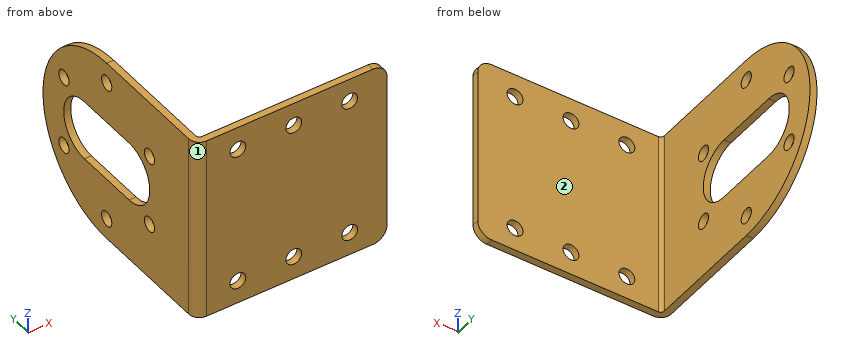
from build123d import *

# Parameters (mm, degrees)
BOSS_EXTRUDE1_DEPTH     = 1.5
SKETCH2_W               = 41
SKETCH2_H               = 40
BOSS_EXTRUDE2_DEPTH     = 1.5
CONVERT_SOLID1_START    = -20
CONVERT_SOLID1_DEPTH    = 40
CONVERT_SOLID1_2_DEPTH  = 40
M3_CLEARANCE_HOLE1_D    = 3.2
CIRPATTERN1_COUNT       = 6
CUT_EXTRUDE1_DEPTH      = 54.525694764
M3_CLEARANCE_HOLE2_D    = 3.4
LPATTERN1_COUNT         = 2
LPATTERN1_PITCH         = 24
LPATTERN1_COPY_1_D      = 3.4
FILLET1_R               = 3
CUT_EXTRUDE2_DEPTH      = 10
CUT_EXTRUDE2_DEPTH_BACK = 66.140233343
SKETCH12_R              = 1.7


# Read off the part's stored shape, not the designer's step: Convert-Solid1
with BuildPart() as part:
    # Sketch1 → Boss-Extrude1 (new body)
    with BuildSketch(Plane(origin=(0, 0, 0), x_dir=(0, 0, -1), z_dir=(1, 0, 0))):
        with BuildLine():
            Line((-20, 0), (-20, -28))
            Line((-20, -28), (20, -28))
            Line((20, -28), (20, 0))
            ThreePointArc((20, 0), (0, 20), (-20, 0))
        make_face()
    extrude(amount=BOSS_EXTRUDE1_DEPTH)

    # Sketch2 → Boss-Extrude2 (add)
    with BuildSketch(Plane.XZ.offset(28)):
        with Locations((20.5, 0)):
            Rectangle(SKETCH2_W, SKETCH2_H)
    extrude(amount=-BOSS_EXTRUDE2_DEPTH)

    # Convert-Solid1 outline → Convert-Solid1 (cut)
    with BuildSketch(Plane.XY.offset(CONVERT_SOLID1_START)):
        with BuildLine():
            Line((0, -28), (2.262, -28))
            ThreePointArc((2.262, -28), (0.662524461, -27.337475539), (0, -25.738))
            Line((0, -25.738), (0, -28))
        make_face()
    extrude(amount=CONVERT_SOLID1_DEPTH, mode=Mode.SUBTRACT)

    # Convert-Solid1 2 outline → Convert-Solid1 2 (add)
    with BuildSketch(Plane.XY.offset(CONVERT_SOLID1_START)):
        with BuildLine():
            Line((1.5, -26.5), (2.262, -26.5))
            ThreePointArc((2.262, -26.5), (1.723184633, -26.276815367), (1.5, -25.738))
            Line((1.5, -25.738), (1.5, -26.5))
        make_face()
    extrude(amount=CONVERT_SOLID1_2_DEPTH)

    # M3 Clearance Hole1 (through all)
    with Locations(Plane.ZY):
        with Locations((-15.5, 0)):
            m3_clearance_hole1 = Hole(M3_CLEARANCE_HOLE1_D / 2)

    # CirPattern1: M3 Clearance Hole1 ×6 about axis
    cirpattern1_axis = Axis((0, 0, 0), (1, 0, 0))
    for i in range(1, CIRPATTERN1_COUNT):
        add(m3_clearance_hole1.rotate(cirpattern1_axis, i * 360 / CIRPATTERN1_COUNT), mode=Mode.SUBTRACT)

    # Sketch9 → Cut-Extrude1 (cut, through all)
    with BuildSketch(Plane.ZY):
        with BuildLine():
            Line((6.5, 7), (6.5, -7))
            ThreePointArc((6.5, -7), (0, -13.5), (-6.5, -7))
            Line((-6.5, -7), (-6.5, 7))
            ThreePointArc((-6.5, 7), (0, 13.5), (6.5, 7))
        make_face()
    extrude(amount=-CUT_EXTRUDE1_DEPTH, mode=Mode.SUBTRACT)

    # M3 Clearance Hole2 (through all)
    with Locations(Plane(origin=(0, -26.5, 0), x_dir=(1, 0, 0), z_dir=(0, 1, 0))):
        with Locations((33, 15)):
            m3_clearance_hole2 = Hole(M3_CLEARANCE_HOLE2_D / 2)

    # Mirror1: M3 Clearance Hole2 across plane
    add(m3_clearance_hole2.mirror(Plane.XY), mode=Mode.SUBTRACT)

    # LPattern1: M3 Clearance Hole2 ×2
    with Locations(*[(-i * LPATTERN1_PITCH, 0, 0) for i in range(1, LPATTERN1_COUNT)]):
        add(m3_clearance_hole2, mode=Mode.SUBTRACT)

    # LPattern1 copy 1 (through all)
    with Locations(Plane(origin=(-24, -26.5, 0), x_dir=(1, 0, 0), z_dir=(0, 1, 0))):
        with Locations((33, -15)):
            Hole(LPATTERN1_COPY_1_D / 2)

    # Fillet1
    fillet1_edges = [part.edges().sort_by_distance(p)[0] for p in [
        (41, -27.25, 20),
        (41, -27.25, -20),
    ]]
    fillet(fillet1_edges, radius=FILLET1_R)

    # Sketch12 → Cut-Extrude2 (cut, two sides: drawn at the far end of the back side and taken through both)
    with BuildSketch(Plane(origin=(0, -26.5, 0), x_dir=(1, 0, 0), z_dir=(0, 1, 0)).offset(-CUT_EXTRUDE2_DEPTH_BACK)):
        with Locations(Location((21, 15, 0), (0, 0, 180))):
            Circle(SKETCH12_R)
        with Locations(Location((21, -15, 0), (0, 0, 180))):
            Circle(SKETCH12_R)
    extrude(amount=CUT_EXTRUDE2_DEPTH + CUT_EXTRUDE2_DEPTH_BACK, mode=Mode.SUBTRACT)


solid = part.part
Work out the finished part from the listing and answer in its coordinate system (mm). Face numbers are marked on the shaded views. A direction names the side the tool comes from. Round coordinates to 2 decimals unless told otherwise and drop trailing zeros. Write each loop counter-clockwise with the first axis right and the second up, starting at its lowest first coordinate (ties: lowest second). Pieces come first, ordered by that corner, then holes. Notation, with made-up numbers: (-18, -3.5) - (11, -3.5) arc R20 ccw to (11, 30.5) - close; hole circle Ø10 at (7, 42.25). An arc over 180 degrees is marked (long way). Answer in a Markdown table with one row per item. Add a question column.
1. A cutting plane is placed at B-B, the plane x = 21. Determine the outline of the cut face in (y, z), and give its area (3 significant figures).
2. Find the intervals of material crossed by line 1 along Z through (x, y) = (9, -27.1); line 2 along X through (y, z) = (-27, -15); line 3 along Y through (x, z) = (21, -17), in increasing order. Write a range as from..to.
3. A cutting plane is placed at A-A, the plane y = -5.5. Determine the outline of the cut face in (x, z).
4. A cutting plane is placed at C-C, the plane z = 2. Determine the outline of the cut face in (x, y), and give its area (3 significant figures).
5. A cutting plane is placed at D-D, the plane y = 4. Determine the outline of the cut face in (x, z).
6. For the marked faces 1 and 2, determine the directions among +Z, -Z, +X, -X, +Y, -Y from which every point of the face is accessible in a straight line to the end or side of a thin tool.
7. Given pin 1 (4.5 mm diameter, centred on x = 33, z = 15, fed in from +Y); pin 2 (1.2 mm diameter, centred on x = 1, y = 2, fed in from +Z); pin 3 (3.5 mm diameter, centred on y = -13.42, z = 7.75, fed in from +X), each flat-ended and moving along its own axis, determine where each tip first touches the part or whether it passes through.
Worked out:
| question | item | result |
|---|---|---|
| 1 | outline | (-28, -20) - (-26.5, -20) - (-26.5, -16.7) - (-28, -16.7) - close; (-28, -13.3) - (-26.5, -13.3) - (-26.5, 13.3) - (-28, 13.3) - close; (-28, 16.7) - (-26.5, 16.7) - (-26.5, 20) - (-28, 20) - close |
| 1 | area | 49.8 mm^2 |
| 2 | line 1 | -20..-16.7, -13.3..13.3, 16.7..20 |
| 2 | line 2 | 0.38..7.3, 10.7..19.3, 22.7..31.3, 34.7..41 |
| 2 | line 3 | -28..-26.5 |
| 3 | outline | (0, -20) - (1.5, -20) - (1.5, -6.5) - (0, -6.5) - close; (0, 6.5) - (1.5, 6.5) - (1.5, 20) - (0, 20) - close |
| 4 | outline | (0, -25.74) arc R2.26 ccw to (2.26, -28) - (41, -28) - (41, -26.5) - (2.26, -26.5) arc R0.76 cw to (1.5, -25.74) - (1.5, -13.18) - (0, -13.18) - close; (0, 13.18) - (1.5, 13.18) - (1.5, 19.9) - (0, 19.9) - close |
| 4 | area | 90.6 mm^2 |
| 5 | outline | (0, -19.6) - (1.5, -19.6) - (1.5, -6.5) - (0, -6.5) - close; (0, 6.5) - (1.5, 6.5) - (1.5, 19.6) - (0, 19.6) - close |
| 6 | face 1 | +Z, -Z, -X, -Y |
| 6 | face 2 | +Z, -Z, +X, +Y |
| 7 | pin 1 | y = -26.5 |
| 7 | pin 2 | z = 19.95 |
| 7 | pin 3 | x = 1.5 |
